```python
from build123d import *
from OCP.BRepFilletAPI import BRepFilletAPI_MakeChamfer

# Parameters (mm, degrees)
BOSS_EXTRUDE1_DEPTH      = 1.5875
BOSS_EXTRUDE1_DEPTH_BACK = 1.5875
SKETCH3_R                = 15.875
SKETCH3_R_2              = 9.5504
CHAMFER1_SIZE            = 0.254
CHAMFER1_SIZE2           = 0.439940905
CHAMFER2_SIZE            = 0.254
CHAMFER2_SIZE2           = 0.495866606


with BuildPart() as part:
    # Sketch3 → Boss-Extrude1 (new, two sides: drawn at the far end of the back side and taken through both)
    with BuildSketch(Plane.XY.offset(-BOSS_EXTRUDE1_DEPTH_BACK)):
        with Locations(Location((0, 0, 0), (0, 0, 180))):
            Circle(SKETCH3_R)
        with Locations(Location((0, 0, 0), (0, 0, 180))):
            Circle(SKETCH3_R_2, mode=Mode.SUBTRACT)
    extrude(amount=BOSS_EXTRUDE1_DEPTH + BOSS_EXTRUDE1_DEPTH_BACK)

    # Chamfer1: one chamfer whose edges measure the first distance from different faces: ONE call of the kernel's chamfer builder (chamfer() names one face for all edges)
    chamfer1_edges_1 = [part.edges().sort_by_distance(p)[0] for p in [
        (15.875, 0, 1.5875),
    ]]
    chamfer1_side_1 = [part.faces().sort_by_distance(p)[0] for p in [
        (15.875, 0, 0.79375),
    ]]
    chamfer1_edges_2 = [part.edges().sort_by_distance(p)[0] for p in [
        (15.875, 0, -1.5875),
    ]]
    chamfer1_side_2 = [part.faces().sort_by_distance(p)[0] for p in [
        (15.875, 0, -0.79375),
    ]]
    chamfer1 = BRepFilletAPI_MakeChamfer(part.part.solid().wrapped)
    for e in chamfer1_edges_1:
        chamfer1.Add(CHAMFER1_SIZE, CHAMFER1_SIZE2, e.wrapped, chamfer1_side_1[0].wrapped)  # the first distance lies on this face
    for e in chamfer1_edges_2:
        chamfer1.Add(CHAMFER1_SIZE, CHAMFER1_SIZE2, e.wrapped, chamfer1_side_2[0].wrapped)  # the first distance lies on this face
    add(Compound.cast(chamfer1.Shape()), mode=Mode.REPLACE)

    # Sketch4 → Cut-Revolve1 (revolve, cut)
    with BuildSketch(Plane(origin=(0, 0, 0), x_dir=(0, 0, -1), z_dir=(1, 0, 0)), mode=Mode.PRIVATE) as cut_revolve1_sk:
        with BuildLine():
            Line((-1.5875, 9.4996), (-1.5875, 9.6012))
            ThreePointArc((-1.5875, 9.6012), (0, 9.5504), (1.5875, 9.6012))
            Line((1.5875, 9.6012), (1.5875, 9.4996))
            Line((1.5875, 9.4996), (-1.5875, 9.4996))
        make_face()
    revolve(cut_revolve1_sk.sketch.rotate(Axis((0, 0, 1.5875), (0, 0, -1)), 180), axis=Axis((0, 0, 1.5875), (0, 0, -1)), mode=Mode.SUBTRACT)

    # Chamfer2: one chamfer whose edges measure the first distance from different faces: ONE call of the kernel's chamfer builder (chamfer() names one face for all edges)
    chamfer2_edges_1 = [part.edges().sort_by_distance(p)[0] for p in [
        (0, 9.6012, -1.5875),
    ]]
    chamfer2_side_1 = [part.faces().sort_by_distance(p)[0] for p in [
        (0, 9.56310325, -0.794156296),
    ]]
    chamfer2_edges_2 = [part.edges().sort_by_distance(p)[0] for p in [
        (0, 9.6012, 1.5875),
    ]]
    chamfer2_side_2 = [part.faces().sort_by_distance(p)[0] for p in [
        (0, 9.56310325, 0.794156296),
    ]]
    chamfer2 = BRepFilletAPI_MakeChamfer(part.part.solid().wrapped)
    for e in chamfer2_edges_1:
        chamfer2.Add(CHAMFER2_SIZE, CHAMFER2_SIZE2, e.wrapped, chamfer2_side_1[0].wrapped)  # the first distance lies on this face
    for e in chamfer2_edges_2:
        chamfer2.Add(CHAMFER2_SIZE, CHAMFER2_SIZE2, e.wrapped, chamfer2_side_2[0].wrapped)  # the first distance lies on this face
    add(Compound.cast(chamfer2.Shape()), mode=Mode.REPLACE)


solid = part.part
```
Work out the finished part from the listing and answer in its coordinate system (mm). Round coordinates to 2 decimals unless told otherwise and drop trailing zeros. Write each loop counter-clockwise with the first axis right and the second up, starting at its lowest first coordinate (ties: lowest second). Pieces come first, ordered by that corner, then holes. Notation, with made-up numbers: (66, -23) - (118, -23) arc R25 cw to (118, 1) - close; hole circle Ø3 at (-5, 40.5). An arc over 180 degrees is marked (long way). Return JSON: item names as keys, results as strings. Group by question number.
Q1. This flat-tipped pin is pushed along its axis until it touches: pin 1 Ø8 at (x, y) = (3, 3) entering from +Z. Where does it stop, or does it pass through?
Q2. The part is cut by section A-A on z = 0.75. Write down the section's boundary in (x, y) (3 decimals), then the cut area to 3 significant figures.
Q3. Find the intervals of material crossed by L1, parallel to X at y = -8.5, z = -0.75; L2, parallel to Y at x = 5, z = 0.1; L3, parallel to Y at x = -4, z = 0.2, in increasing order.
Solved:
{
 "1": {"pin 1": "through"},
 "2": {"outline": "circle Ø31.75 at (0, 0); hole circle Ø19.123 at (0, 0)", "area": "505 mm²"},
 "3": {"L1": "-13.41 to -4.38, 4.38 to 13.41", "L2": "-15.07 to -8.14, 8.14 to 15.07", "L3": "-15.36 to -8.67, 8.67 to 15.36"}
}
